Autodesk Inventor part; units mm, degrees
ref_plane "Work Plane1" through (6.5151, 0, 0) normal (1, 0, 0) x (0, 1, 0)
ref_plane "Work Plane2" through (0, -8.6106, 0) normal (0, 1, 0) x (-1, 0, 0)
ref_plane "XY Plane" through (0, 0, 0) normal (0, 0, 1) x (1, 0, 0)
ref_plane "Work Plane1" through (6.5151, 0, 0) normal (1, 0, 0) x (0, 1, 0)
sketch "Sketch2" plane through (0, 0, 0) normal (0, 0, 1) x (1, 0, 0)
  circle A0 centre (0, 0) radius 8.636
  circle A1 centre (0, 0) radius 4.5212
  line L0 (0, -8.636) -> (0, -27.432) construction
  dimension "d2" = 17.272
  dimension "d3" = 4.1148
  dimension "d4" = 18.796
extrude "Extrusion1" add sketch "Sketch2" along normal mid plane 4.318
ref_plane "Work Plane2" through (0, -8.6106, 0) normal (0, 1, 0) x (-1, 0, 0)
sketch "Sketch3" plane through (0, -8.6106, 0) normal (0, 1, 0) x (-1, 0, 0)
  circle A0 centre (0, 0) radius 2.0574
  dimension "d8" = 4.1148
extrude "Extrusion2" add sketch "Sketch3" against normal blind 18.796
properties part number "eye screw stand-in"
Part model, mm, in its own coordinate system. A direction names the side the tool comes from. Coordinates: 2 decimals unless noted, no trailing zeros. Loops run counter-clockwise (first coordinate to the right, second up) from the corner with the lowest first, then second, coordinate; pieces in that order, holes last. Notation, with made-up numbers: (50, 13) - (60, 13) arc R25 ccw to (60, 46) - close; hole circle Ø10 at (4, 54.25). An arc over 180 degrees is marked (long way). Write each question's results on one line, items separated by ' | '. Start each with the question number.
Q1. Drop flat-ended pins along their axis: pin 1 Ø0.7 at (x, z) = (-1.5, 1) entering from +Y; pin 2 Ø7 at (x, y) = (0, 0) entering from +Z; pin 3 Ø4 at (x, y) = (-0.5, -13) entering from -Z. Give the stop position or say it passes through.
Q2. Slice it at C-C on z = 0. Give the cut face in (x, y), and give its area (3 significant figures).
Q3. Slice it at D-D on x = -4. Give the cut face in (y, z), and give its area (3 significant figures).
Q4. Which spindle directions (+Z, -Z, +X, -X, +Y, -Y) get a long thin tool onto all of the face, cutting with end or side? Do faces 1 (the cylindrical face through (2.055, -17.877, 0.09)), 2 (the flat face through (4, -4, -2.159)). Say none if no direction does.
Q5. Slice it at A-A on y = 0. Give the cut face in (x, z).
Q6. Probe line 1 along Y through (x, z) = (0, 0.2); line 2 along X through (y, z) = (4, -2); line 3 along Z through (x, y) = (0, -22). List the from-to ranges inside material, lowest first.
Q7. Slice it at B-B on x = 0. Give the cut face in (y, z), and give its area (3 significant figures).
Answer:
1) pin 1: stops at y = 8.56 | pin 2: passes through | pin 3: stops at z = -2.06
2) outline: (-2.06, -27.41) - (2.06, -27.41) - (2.06, -8.61) - (0.66, -8.61) arc R8.64 ccw (long way) to (-0.66, -8.61) - (-2.06, -8.61) - close; hole circle Ø9.04 at (0, 0) | area: 247 mm2
3) outline: (-7.65, -2.16) - (-2.11, -2.16) - (-2.11, 2.16) - (-7.65, 2.16) - close; (2.11, -2.16) - (7.65, -2.16) - (7.65, 2.16) - (2.11, 2.16) - close | area: 47.9 mm2
4) face 1: -Y | face 2: -Z, +X, -X, +Y, -Y
5) outline: (-8.64, -2.16) - (-4.52, -2.16) - (-4.52, 2.16) - (-8.64, 2.16) - close; (4.52, -2.16) - (8.64, -2.16) - (8.64, 2.16) - (4.52, 2.16) - close
6) line 1: y = -27.41 to -4.52, 4.52 to 8.64 | line 2: x = -7.65 to -2.11, 2.11 to 7.65 | line 3: z = -2.06 to 2.06
7) outline: (-27.41, -2.06) - (-8.64, -2.06) - (-8.64, -2.16) - (-4.52, -2.16) - (-4.52, 2.16) - (-8.64, 2.16) - (-8.64, 2.06) - (-27.41, 2.06) - close; (4.52, -2.16) - (8.64, -2.16) - (8.64, 2.16) - (4.52, 2.16) - close | area: 113 mm2
